Here's how the part is built. I have some questions about the finished solid (model axes, mm). A direction names the side the tool comes from. Round coordinates to 2 decimals unless told otherwise and drop trailing zeros. Order: outer loops, then holes, each group sorted by start corner. A loop starts at its lowest first (then second) coordinate and runs counter-clockwise, first axis right, second up. Notation, with made-up numbers: (26.5, 5) -> (82.5, 5) arc R27 ccw to (82.5, 29) -> close; hole circle Ø2 at (82.25, 57.5). An arc over 180 degrees is marked (long way). One line per item, written item: value.
```python
from build123d import *

# Parameters (mm, degrees)
CHAMFER_SIZE    = 0.25
CHAMFER001_SIZE = 0.1
CHAMFER002_SIZE = 0.1


with BuildPart() as part:
    # Sketch003 → Revolution003 (revolve)
    with BuildSketch(Plane.XZ):
        Polygon((2.5, 31), (3.49, 30.01), (3.49, 29.35), (2.815, 29), (2.815, 27.5), (3.49, 27.15), (3.49, 24), (5, 24), (5, 13.6), (1.25, 13.6), (1.25, 27.849785), (1.5, 28), (1.5, 31), align=None)
    revolve(axis=Axis((0, 0, 0), (0, 0, 1)))

    # Chamfer
    chamfer_edges = [part.edges().sort_by_distance(p)[0] for p in [
        (-5, 0, 13.6),
    ]]
    chamfer(chamfer_edges, length=CHAMFER_SIZE)

    # Chamfer001
    chamfer001_edges = [part.edges().sort_by_distance(p)[0] for p in [
        (-2.815, 0, 29),
    ]]
    chamfer(chamfer001_edges, length=CHAMFER001_SIZE)

    # Chamfer002
    chamfer002_edges = [part.edges().sort_by_distance(p)[0] for p in [
        (-3.49, 0, 24),
    ]]
    chamfer(chamfer002_edges, length=CHAMFER002_SIZE)


solid = part.part
```
Q1. For P1, Ø2, axis at y = 1.5, z = 21.5, coming from the -X side, with a flat end and sliding along its axis, tell me the tip position at first contact or that it passes through.
Answers:
P1: x = -4.97
Q2. If we mould it in two halves opening along Y, with no side actions, what happens to faces 1 (the face through (-0.27, -1.22, 20.82)), 2 (the face through (1, -1, 13.6)), 3 (the face through (-1.08, -4.88, 18.85))? For each: pulls with the +Y half, pulls with the -Y half, needs draft (parallel to the pull), parting line crosses it, or undercut.
Answers:
face 1: undercut
face 2: needs draft
face 3: parting line crosses it
Q3. I need wall thicknesses on line 1 along Y through (x, z) = (0, 17.5); line 2 along Y through (x, z) = (0, 30); line 3 along Z through (x, y) = (1.5, 3.5). Which ranges of each line are inside material? Lowest first, please.
Answers:
line 1: -5 to -1.25, 1.25 to 5
line 2: -3.49 to -1.5, 1.5 to 3.49
line 3: 13.6 to 24
Q4. Which directions (+Z, -Z, +X, -X, +Y, -Y) give clear straight access to the entire face, cutting with the end or side of a thin tool? Please do faces 4 (the face through (-2, 0, 31)), 5 (the face through (2.7, 0.8, 28.2)), 6 (the face through (-0.45, 3.46, 29.68)).
Answers:
face 4: +Z, +X, -X, +Y, -Y
face 5: none
face 6: +Z
Q5. I want a section at A-A on z = 15.25. Write out the boundary of the cut face in (x, y).
Answers:
outline: circle Ø10 at (0, 0); hole circle Ø2.5 at (0, 0)
Q6. I want a section at B-B on z = 26. Write out the boundary of the cut face in (x, y).
Answers:
outline: circle Ø6.98 at (0, 0); hole circle Ø2.5 at (0, 0)
